from build123d import *

# Parameters (mm, degrees)
SKETCH1_W           = 10
SKETCH1_H           = 10
BOSS_EXTRUDE1_DEPTH = 3
SKETCH2_W           = 10
SKETCH2_H           = 8
BOSS_EXTRUDE2_DEPTH = 12
SKETCH3_W           = 6.2
SKETCH3_H           = 9
CUT_EXTRUDE1_DEPTH  = 5.8
SKETCH4_R           = 0.75
CUT_EXTRUDE2_DEPTH  = 20.64281039


with BuildPart() as part:
    # Sketch1 → Boss-Extrude1 (new body)
    with BuildSketch(Plane(origin=(0, 0, 0), x_dir=(1, 0, 0), z_dir=(0, 1, 0))):
        with Locations((5, 5)):
            Rectangle(SKETCH1_W, SKETCH1_H)
    extrude(amount=BOSS_EXTRUDE1_DEPTH)

    # Sketch2 → Boss-Extrude2 (add)
    with BuildSketch(Plane(origin=(0, 3, 0), x_dir=(1, 0, 0), z_dir=(0, 1, 0))):
        with Locations((5, 6)):
            Rectangle(SKETCH2_W, SKETCH2_H)
    extrude(amount=BOSS_EXTRUDE2_DEPTH)

    # Sketch3 → Cut-Extrude1 (cut)
    with BuildSketch(Plane.XY.offset(-2)):
        with Locations((5, 7.5)):
            Rectangle(SKETCH3_W, SKETCH3_H)
    extrude(amount=-CUT_EXTRUDE1_DEPTH, mode=Mode.SUBTRACT)

    # Sketch4 → Cut-Extrude2 (cut, through all)
    with BuildSketch(Plane.XY.offset(-7.8)):
        with Locations((5, 9.3)):
            Circle(SKETCH4_R)
    extrude(amount=-CUT_EXTRUDE2_DEPTH, mode=Mode.SUBTRACT)


solid = part.part
The listing builds one solid part. Answer for the finished solid, in the listing's coordinates (mm). A direction names the side the tool comes from. Give positions to 0.01 mm unless a question says otherwise; leave off trailing zeros. Loops run counter-clockwise (first coordinate to the right, second up) from the corner with the lowest first, then second, coordinate; pieces in that order, holes last. Notation, with made-up numbers: (10.5, 59.25) - (23.5, 59.25) arc R10 cw to (23.5, 68.25) - close; hole circle Ø8 at (-29.75, 55). An arc over 180 degrees is marked (long way). Use one line per item in the form item = value.
1. Section C-C on z = -3 is taken. Give the vertices of the cut face in (x, y), then the cut area to 3 significant figures.
Calculated:
outline = (0, 0) - (10, 0) - (10, 15) - (0, 15) - close; hole (1.9, 3) - (8.1, 3) - (8.1, 12) - (1.9, 12) - close
area = 94.2 mm^2
2. Section B-B on y = 9.3 is taken. Give the vertices of the cut face in (x, z).
Calculated:
outline = (0, -10) - (4.25, -10) - (4.25, -7.8) - (1.9, -7.8) - (1.9, -2) - (0, -2) - close; (5.75, -10) - (10, -10) - (10, -2) - (8.1, -2) - (8.1, -7.8) - (5.75, -7.8) - close
3. Section A-A on x = 5 is taken. Give the vertices of the cut face in (y, z).
Calculated:
outline = (0, -10) - (8.55, -10) - (8.55, -7.8) - (3, -7.8) - (3, 0) - (0, 0) - close; (10.05, -10) - (15, -10) - (15, -2) - (12, -2) - (12, -7.8) - (10.05, -7.8) - close
4. Find the intervals of material crossed by line 1 along Y through (x, z) = (5, -8.85); line 2 along X through (y, z) = (10.25, -3.25); line 3 along Y through (x, z) = (2, -4.5), in increasing order. Write a range as [from, to].
Calculated:
line_1 = [0, 8.55], [10.05, 15]
line_2 = [0, 1.9], [8.1, 10]
line_3 = [0, 3], [12, 15]
5. Given pin 1 Ø1.7 at (x, y) = (5, 9.3) entering from +Z; pin 2 Ø6 at (x, y) = (3.5, 11) entering from +Z, each flat-ended and moving along its own axis, determine where each tip first touches the part or whether it passes through.
Calculated:
pin_1 = -7.8
pin_2 = -2
6. Which of the six approach directions +Z, -Z, +X, -X, +Y, -Y give full straight-line access (tool end or side, diameter ignored) to faces 4 (the face through (5, 1, 0)), 5 (the face through (5, 8, -7.8)), 6 (the face through (5, 13, -2))?
Calculated:
face_4 = +Z, +X, -X, +Y, -Y
face_5 = +Z
face_6 = +Z, +X, -X, +Y
7. Section D-D on x = 6 is taken. Give the vertices of the cut face in (y, z).
Calculated:
outline = (0, -10) - (15, -10) - (15, -2) - (12, -2) - (12, -7.8) - (3, -7.8) - (3, 0) - (0, 0) - close
8. The mould has two halves that part along X. Classify faces 1 (the face through (5, 15, -6)), 2 (the face through (1.9, 7, -5)), 3 (the face through (10, 7, -6)): pulls with the +X half, pulls with the -X half, needs draft (parallel to the pull), parting line crosses it, or undercut.
Calculated:
face_1 = needs draft
face_2 = undercut
face_3 = pulls with the +X half
